```python
from build123d import *

# Parameters (mm, degrees)
F2_R     = 2
F3_SIZE  = 0.5
F4_R     = 6.25
F5_DEPTH = 20.1
F6_SIZE  = 1


with BuildPart() as f1:
    # F0 (on Front) → F1 (revolve)
    with BuildSketch(Plane.XZ):
        Polygon((-6, 0), (0, 0), (0, 145), (-11, 145), (-11, 120), (-8, 120), (-8, 13.25), (-6, 13.25), (-6, 7.5), (-2.75, 7.5), (-2.75, 3), (-6, 3), align=None)
    revolve(axis=Axis((0, 0, 49.5666371724), (0, 0, 1)))

    # F2
    f2_edges = [f1.edges().sort_by_distance(p)[0] for p in [
        (2.75, 0, 7.5),
        (2.75, 0, 3),
        (-2.75, 0, 5.25),
    ]]
    fillet(f2_edges, radius=F2_R)

    # F3
    f3_edges = [f1.edges().sort_by_distance(p)[0] for p in [
        (6, 0, 7.5),
        (6, 0, 3),
        (6, 0, 0),
    ]]
    chamfer(f3_edges, length=F3_SIZE)

    # F4 (on Right) → F5 (cut, symmetric)
    with BuildSketch(Plane.YZ):
        with Locations((0, 132.5)):
            Circle(F4_R)
    extrude(amount=F5_DEPTH, both=True, mode=Mode.SUBTRACT)

    # F6
    f6_edges = [f1.edges().sort_by_distance(p)[0] for p in [
        (11, 0, 145),
        (11, 0, 120),
    ]]
    chamfer(f6_edges, length=F6_SIZE)


solid = f1.part
```
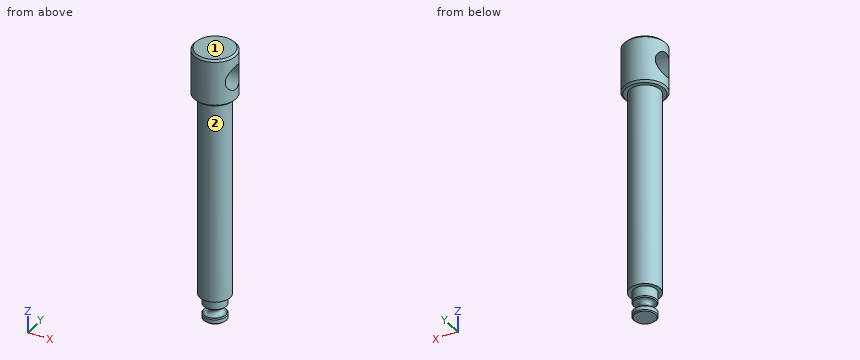
Work out the finished part from the listing and answer in its coordinate system (mm). Face numbers are marked on the shaded views. A direction names the side the tool comes from. Round coordinates to 2 decimals unless told otherwise and drop trailing zeros. Loops run counter-clockwise (first coordinate to the right, second up) from the corner with the lowest first, then second, coordinate; pieces in that order, holes last.
(1) Each of these flat-tipped pins is pushed along its axis until it touches: P1, Ø8, axis at x = -8.5, z = 123, coming from the -Y side; P2, Ø12, axis at x = 1.5, z = 49.5, coming from the +Y side; P3, Ø3, axis at x = 5, z = 44, coming from the -Y side. Where does it stop, or does it pass through?
Computed values:
P1: stops at y = -10.04
P2: stops at y = 8
P3: stops at y = -7.19
(2) The part is cut by section B-B, the plane z = 135.5. Give the vertices of the cut face in (x, y).
Computed values:
outline: (-9.54, -5.48) arc R11 ccw to (9.54, -5.48) - close; (-9.54, 5.48) - (9.54, 5.48) arc R11 ccw to start
(3) The part is cut by section C-C, the plane z = 62.5. Give the vertices of the cut face in (x, y), and give its area (3 significant figures).
Computed values:
outline: circle Ø16 at (0, 0)
area: 201 mm2
(4) Find the intervals of material crossed by L1, parallel to Z at x = -5, y = 0; L2, parallel to Z at x = -4, y = 0; L3, parallel to Z at x = 1.25, y = -1.25, in increasing order.
Computed values:
L1: z = 0 to 3, 7.5 to 126.25, 138.75 to 145
L2: z = 0 to 3.15, 7.35 to 126.25, 138.75 to 145
L3: z = 0 to 126.38, 138.62 to 145
(5) The part is cut by section A-A, the plane z = 12. Give the vertices of the cut face in (x, y).
Computed values:
outline: circle Ø12 at (0, 0)
(6) For the marked faces 1 and 2, determine the directions among +Z, -Z, +X, -X, +Y, -Y from which every point of the face is accessible in a straight line to the end or side of a thin tool.
Computed values:
face 1: +Z, +X, -X, +Y, -Y
face 2: -Z
